```python
from build123d import *

# Parameters (mm, degrees)
F0_W     = 203.2
F0_H     = 203.2
F0_R     = 3.175
F1_DEPTH = 19.304
F2_R     = 5.08
F4_DEPTH = 14.224
F5_D     = 4.9
F5_DEPTH = 12
F5_TIP   = 1.4721085166


with BuildPart() as f1:
    # F0 (on Top) → F1 (new body)
    with BuildSketch(Plane.XY):
        Rectangle(F0_W, F0_H)
        with Locations((-88.9, -88.9)):
            Circle(F0_R, mode=Mode.SUBTRACT)
        with Locations((88.9, -88.9)):
            Circle(F0_R, mode=Mode.SUBTRACT)
        with Locations((0, 19.05)):
            Circle(F0_R, mode=Mode.SUBTRACT)
        with Locations((-88.9, 88.9)):
            Circle(F0_R, mode=Mode.SUBTRACT)
        with Locations((88.9, 88.9)):
            Circle(F0_R, mode=Mode.SUBTRACT)
    extrude(amount=F1_DEPTH)

    # F2 (on face) → F4 (cut, through all)
    with BuildSketch(Plane.XY.offset(19.304)):
        with Locations((-88.9, 88.9)):
            Circle(F2_R)
        with Locations((0, 19.05)):
            Circle(F2_R)
        with Locations((88.9, 88.9)):
            Circle(F2_R)
        with Locations((-88.9, -88.9)):
            Circle(F2_R)
        with Locations((88.9, -88.9)):
            Circle(F2_R)
    extrude(amount=-F4_DEPTH, mode=Mode.SUBTRACT)

    # F5
    with Locations(Plane.XY.offset(19.304)):
        with Locations((0, -88.9), (88.9, 0), (0, 88.9), (-88.9, 0), (-88.9, -71.12), (-71.12, -88.9), (-88.9, 71.12), (-71.12, 88.9), (71.12, 88.9), (88.9, 71.12), (88.9, -71.12), (71.12, -88.9)):
            Hole(F5_D / 2, depth=F5_DEPTH)
            with Locations((0, 0, -(F5_DEPTH + F5_TIP / 2))):  # 118° drill point
                Cone(0, F5_D / 2, F5_TIP, mode=Mode.SUBTRACT)


solid = f1.part
```
Check sheet for the modelled part. Datum: model origin and axes. Units: mm. A direction names the side the tool comes from. Coordinates: 2 decimals unless noted, no trailing zeros. Use one line per item in the form item = value.
Item 1: Gauge pin test, flat ends, axial feed: pin 1 Ø4.5 at (x, y) = (-88.9, 71.12) entering from +Z; pin 2 Ø7.5 at (x, y) = (0, 19.05) entering from -Z; pin 3 Ø5 at (x, y) = (-90, 87.5) entering from +Z; pin 4 Ø4 at (x, y) = (0, -88.9) entering from +Z. Record the tip position at first contact, or that the pin passes through.
Answer below:
pin_1 = 7.18
pin_2 = 0
pin_3 = 5.08
pin_4 = 7.03
Item 2: Sectioned sample at A-A, the plane z = 13. State how many separate pieces and enclosed holes the cut face has, and give its area (3 significant figures).
Answer below:
separate_pieces = 1
enclosed_holes = 17
area = 40,700 mm^2
Item 3: Material ranges on L1, parallel to Y at x = -89, z = 14; L2, parallel to X at y = 71.12, z = 11.5, recorded low to high. Write a range as from..to.
Answer below:
L1 = -101.6..-93.98, -83.82..-73.57, -68.67..-2.45, 2.45..68.67, 73.57..83.82, 93.98..101.6
L2 = -101.6..-91.35, -86.45..86.45, 91.35..101.6
Item 4: Set-up check for faces 1 (the face through (-86.56, -93.41, 12.29)), 2 (the face through (-1, 101.6, 10)): record each of +Z, -Z, +X, -X, +Y, -Y from which the full face is reachable in a straight line by a thin tool's end or side.
Answer below:
face_1 = +Z
face_2 = +Z, -Z, +X, -X, +Y
Item 5: Release check for a two-part mould opening along X. For faces 3 (the face through (-1, 1, 19.304)), 4 (the face through (89.1, -71.5, 6.09)), 5 (the face through (101.6, -1, 10)) record: pulls with the +X half, pulls with the -X half, needs draft (parallel to the pull), parting line crosses it, or undercut.
Answer below:
face_3 = needs draft
face_4 = undercut
face_5 = pulls with the +X half
